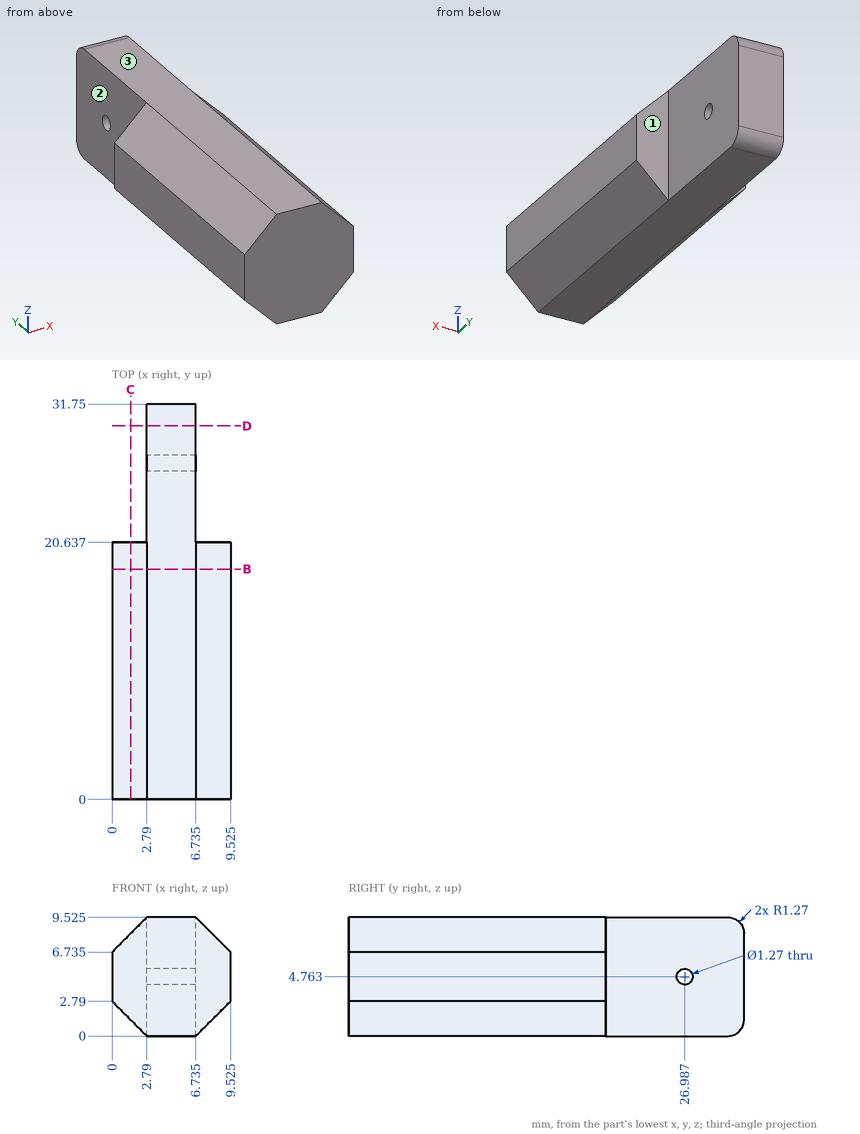
Verification items for this drawing (mm, ordinates from the low corner). A direction names the side the tool comes from. Coordinates: 2 decimals unless noted, no trailing zeros. Write each loop counter-clockwise with the first axis right and the second up, starting at its lowest first coordinate (ties: lowest second). Pieces come first, ordered by that corner, then holes. Notation, with made-up numbers: M 8,37 L 18,37 A32 ccw 18,70 Z; hole C 58,10.25 d1. An arc over 180 degrees is marked long. Answer as a JSON object with one key per item and string values. Group by question number.
(1) Tool access check on the marked faces 1, 2 and 3. Record the directions out of +Z, -Z, +X, -X, +Y, -Y that give a thin tool (end or side, any length) a straight path to the whole face; none if there is none.
(2) Material ranges on line 1 (X direction, y = 23.5, z = 9.25) (1 decimal); line 2 (Y direction, x = 2.5, z = 5); line 3 (X direction, y = 15, z = 1) (1 decimal), recorded low to high.
(3) Gauge pin test, flat ends, axial feed: pin 1 (1.5 mm diameter, centred on y = 26.99, z = 4.76, fed in from -X); pin 2 (0.8 mm diameter, centred on x = 1.5, z = 5.5, fed in from +Y); pin 3 (5 mm diameter, centred on y = 23.5, z = 5.5, fed in from +X) (1 decimal). Record the tip position at first contact, or that the pin passes through.
(4) Cross-section at B-B, the plane y = 18.5. Record the cut outline in (x, z) (1 decimal).
(5) Cross-section at C-C, the plane x = 1.5. Record the cut outline in (y, z) (1 decimal), and give its area (3 significant figures).
(6) Cross-section at D-D, the plane y = 30. Record the cut outline in (x, z) (1 decimal).
Reply:
{
 "1": {"face 1": "+Z, -Z, +X, +Y", "face 2": "+Z, -Z, -X, +Y", "face 3": "+Z, +X, -X, +Y, -Y"},
 "2": {"line 1": "2.8 to 6.7", "line 2": "0 to 20.64", "line 3": "1.8 to 7.7"},
 "3": {"pin 1": "x = 2.79", "pin 2": "y = 20.64", "pin 3": "x = 6.7"},
 "4": {"outline": "M 0,2.8 L 2.8,0 L 6.7,0 L 9.5,2.8 L 9.5,6.7 L 6.7,9.5 L 2.8,9.5 L 0,6.7 Z"},
 "5": {"outline": "M 0,1.3 L 20.6,1.3 L 20.6,8.2 L 0,8.2 Z", "area": "143 mm²"},
 "6": {"outline": "M 2.8,0 L 6.7,0 L 6.7,9.5 L 2.8,9.5 Z"}
}
